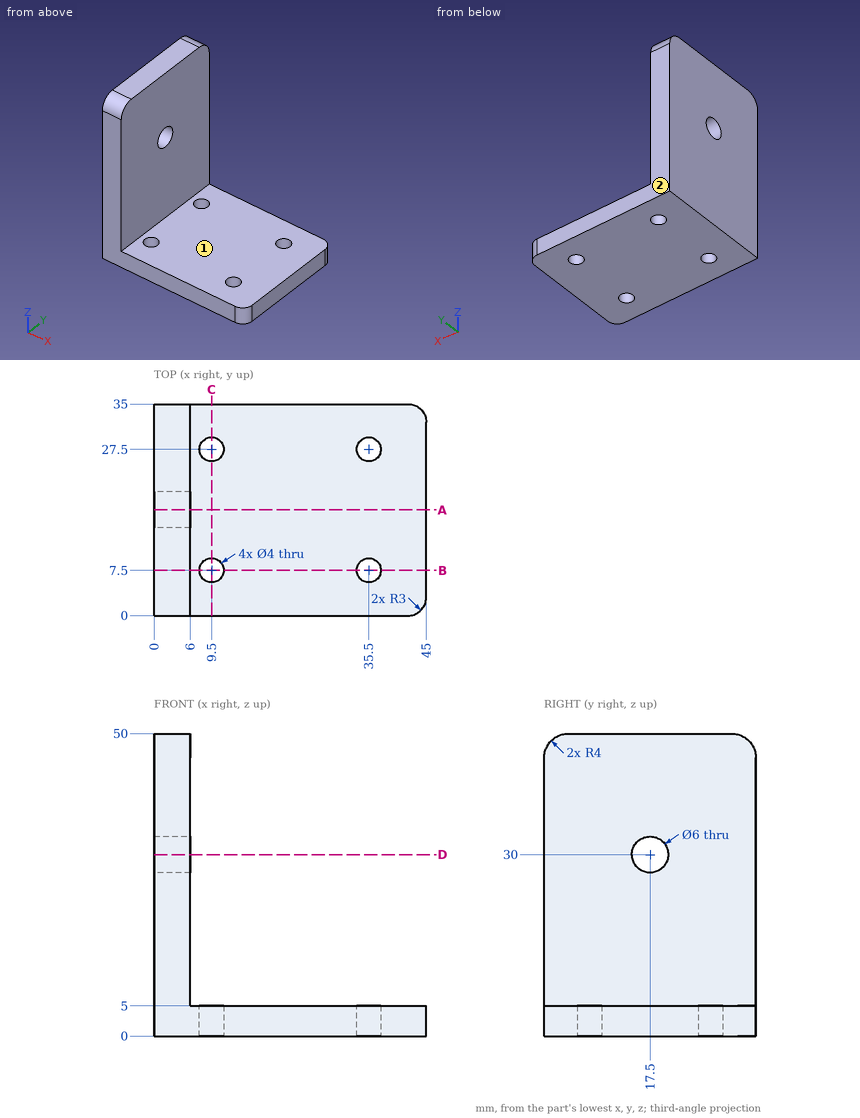
Geometry: see drawing. Coordinates: mm, zero at the bounding-box minimum. A direction names the side the tool comes from. Give positions to 0.01 mm unless a question says otherwise; leave off trailing zeros. Write each loop counter-clockwise with the first axis right and the second up, starting at its lowest first coordinate (ties: lowest second). Pieces come first, ordered by that corner, then holes. Notation, with made-up numbers: (28, 16) - (34, 16) arc R29 cw to (34, 47) - close; hole circle Ø1 at (55.5, -13). An arc over 180 degrees is marked (long way). Return JSON: item names as keys, results as strings. Group by question number.
1) Section A-A on y = 17.5. Return the cut outline in (x, z).
2) Section C-C on x = 9.5. Return the cut outline in (y, z).
3) Set-up query: the marked faces 1 and 2. Return all of +Z, -Z, +X, -X, +Y, -Y with unobstructed straight access to the full face (end or side cutting, diameter ignored); none if empty.
4) Section D-D on z = 30. Return the cut outline in (x, y), plus the area to 3 significant figures.
5) Line query: line 1 (Y direction, x = 9.5, z = 1.6); line 2 (Y direction, x = 3.2, z = 30); line 3 (Y direction, x = 8.5, z = 4). Output: solid intervals per line, ascending.
6) First-contact query: P1, Ø3.5, axis at x = 35.5, y = 7.5, coming from the +Z side; P2, Ø5, axis at y = 16.5, z = 11, coming from the +X side; P3, Ø3, axis at x = 31, y = 23, coming from the +Z side. Flat tips, straight axial feed; report the tip coordinate or a pass-through.
7) Section B-B on y = 7.5. Return the cut outline in (x, z), plus the area to 3 significant figures.
Filled in:
{
 "1": {"outline": "(0, 0) - (45, 0) - (45, 5) - (6, 5) - (6, 27) - (0, 27) - close; (0, 33) - (6, 33) - (6, 50) - (0, 50) - close"},
 "2": {"outline": "(0, 0) - (5.5, 0) - (5.5, 5) - (0, 5) - close; (9.5, 0) - (25.5, 0) - (25.5, 5) - (9.5, 5) - close; (29.5, 0) - (35, 0) - (35, 5) - (29.5, 5) - close"},
 "3": {"face 1": "+Z, +X, +Y, -Y", "face 2": "+Z, -Z, +X, -X, +Y"},
 "4": {"outline": "(0, 0) - (6, 0) - (6, 14.5) - (0, 14.5) - close; (0, 20.5) - (6, 20.5) - (6, 35) - (0, 35) - close", "area": "174 mm^2"},
 "5": {"line 1": "y = 0 to 5.5, 9.5 to 25.5, 29.5 to 35", "line 2": "y = 0 to 14.5, 20.5 to 35", "line 3": "y = 0 to 5.77, 9.23 to 25.77, 29.23 to 35"},
 "6": {"P1": "passes through", "P2": "stops at x = 6", "P3": "stops at z = 5"},
 "7": {"outline": "(0, 0) - (7.5, 0) - (7.5, 5) - (6, 5) - (6, 50) - (0, 50) - close; (11.5, 0) - (33.5, 0) - (33.5, 5) - (11.5, 5) - close; (37.5, 0) - (45, 0) - (45, 5) - (37.5, 5) - close", "area": "455 mm^2"}
}
